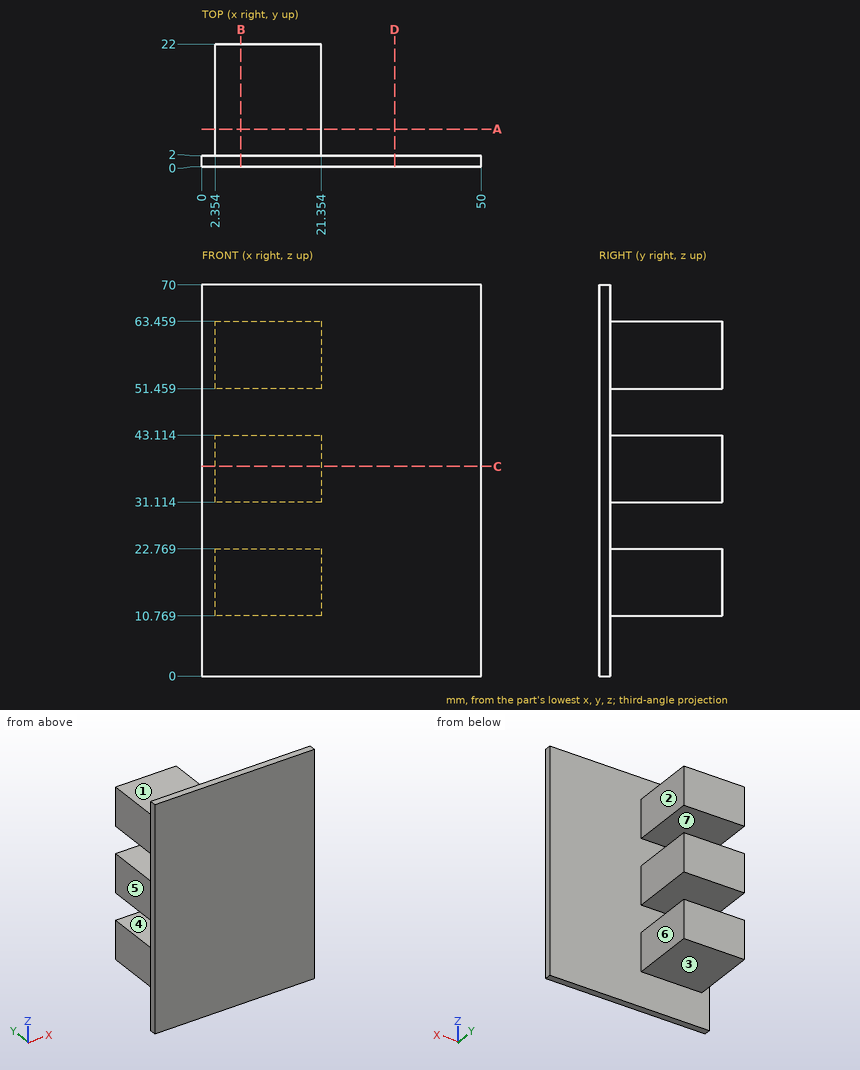
Could you check a few things on this drawing? It's one solid part, dimensions in mm from its lowest x, y, z. A direction names the side the tool comes from. Round coordinates to 2 decimals unless told otherwise and drop trailing zeros. Loops run counter-clockwise (first coordinate to the right, second up) from the corner with the lowest first, then second, coordinate; pieces in that order, holes last. Notation, with made-up numbers: (26.25, 81.5) -> (66.25, 81.5) arc R24 ccw to (66.25, 92.5) -> close; hole circle Ø5 at (29, 39). An arc over 180 degrees is marked (long way). One line per item, written item: value. Start each with the question number.
1. If we section it at C-C, the plane z = 37.5: Write out the boundary of the cut face in (x, y) (1 decimal).
2. If we mould it in two halves opening along Z, with no side actions, what happens to the marked faces 1, 2, 3 and 4? For each: pulls with the +Z half, pulls with the -Z half, needs draft (parallel to the pull), parting line crosses it, or undercut.
3. For the marked faces 5, 6 and 7, which set-ups out of +Z, -Z, +X, -X, +Y, -Y let a thin tool reach every point of the face, with its end or its side?
4. If we section it at B-B, the plane x = 7: Write out the boundary of the cut face in (y, z), then the cut area to 3 significant figures.
5. If we section it at A-A, the plane y = 6.75: Write out the boundary of the cut face in (x, z) (1 decimal), then the cut area to 3 significant figures.
6. If we section it at D-D, the plane x = 34.5: Write out the boundary of the cut face in (y, z).
7. For pin 1 (13 mm diameter, centred on y = 14.5, z = 17.5, fed in from -X); pin 2 (9.5 mm diameter, centred on x = 13.5, y = 7, fed in from +Z); pin 3 (1 mm diameter, centred on y = 19, z = 39, fed in from +X), each with a flat end and sliding along its axis, tell me the tip position at first contact or that it passes through.
8. If I drill on probe 1 along Z at (x, y) = (3, 6); probe 2 along Y at (x, z) = (11, 5.5); probe 3 along X at (y, z) = (4.25, 62) (1 decimal), over which ranges is the centre line in solid material (lowest first)?
Calculated:
1. outline: (0, 0) -> (50, 0) -> (50, 2) -> (21.4, 2) -> (21.4, 22) -> (2.4, 22) -> (2.4, 2) -> (0, 2) -> close
2. face 1: pulls with the +Z half
2. face 2: needs draft
2. face 3: pulls with the -Z half
2. face 4: undercut
3. face 5: +Z, -Z, -X, +Y
3. face 6: +Z, -Z, +X, +Y
3. face 7: +X, -X, +Y
4. outline: (0, 0) -> (2, 0) -> (2, 10.77) -> (22, 10.77) -> (22, 22.77) -> (2, 22.77) -> (2, 31.11) -> (22, 31.11) -> (22, 43.11) -> (2, 43.11) -> (2, 51.46) -> (22, 51.46) -> (22, 63.46) -> (2, 63.46) -> (2, 70) -> (0, 70) -> close
4. area: 860 mm²
5. outline: (2.4, 10.8) -> (21.4, 10.8) -> (21.4, 22.8) -> (2.4, 22.8) -> close; (2.4, 31.1) -> (21.4, 31.1) -> (21.4, 43.1) -> (2.4, 43.1) -> close; (2.4, 51.5) -> (21.4, 51.5) -> (21.4, 63.5) -> (2.4, 63.5) -> close
5. area: 684 mm²
6. outline: (0, 0) -> (2, 0) -> (2, 70) -> (0, 70) -> close
7. pin 1: stops at x = 2.35
7. pin 2: stops at z = 63.46
7. pin 3: stops at x = 21.35
8. probe 1: z = 10.77 to 22.77, 31.11 to 43.11, 51.46 to 63.46
8. probe 2: y = 0 to 2
8. probe 3: x = 2.4 to 21.4
